Design review of the part built by this model. Coordinates are the model's own, in mm. Coordinates: 2 decimals unless noted, no trailing zeros. Loops run counter-clockwise (first coordinate to the right, second up) from the corner with the lowest first, then second, coordinate; pieces in that order, holes last. Notation, with made-up numbers: M 12,89 L 21,89 A19 cw 21,112 Z; hole C 37.5,-6.75 d8. An arc over 180 degrees is marked long. Write item = value, one per line. Start each with the question number.
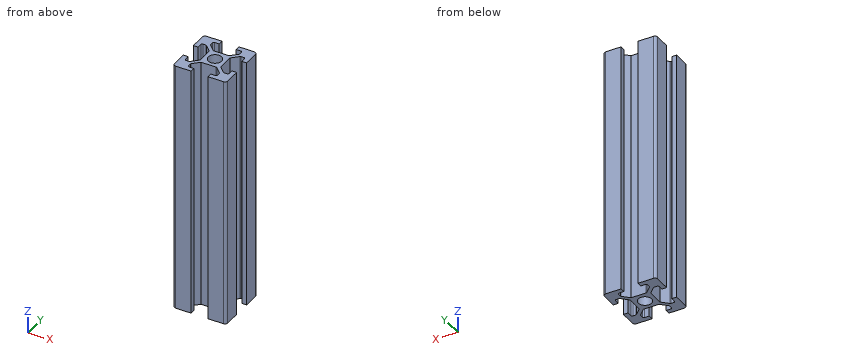
```python
from build123d import *

# Parameters (mm, degrees)
SKETCH1_R           = 2.5
BOSS_EXTRUDE1_DEPTH = 95
FILLET1_R           = 1
FILLET2_R           = 0.5
FILLET3_R           = 0.5
FILLET4_R           = 0.5
FILLET5_R           = 0.5


with BuildPart() as part:
    # Sketch1 → Boss-Extrude1 (new body)
    with BuildSketch(Plane.XY):
        Polygon((13.2, 0), (13.2, 1.8), (15.45, 1.8), (15.45, 3.6), (12.95, 6.1), (7.05, 6.1), (4.55, 3.6), (4.55, 1.8), (6.8, 1.8), (6.8, 0), (0, 0), (0, 6.8), (1.8, 6.8), (1.8, 4.55), (3.6, 4.55), (6.1, 7.05), (6.1, 12.95), (3.6, 15.45), (1.8, 15.45), (1.8, 13.2), (0, 13.2), (0, 20), (6.8, 20), (6.8, 18.2), (4.55, 18.2), (4.55, 16.4), (7.05, 13.9), (12.95, 13.9), (15.45, 16.4), (15.45, 18.2), (13.2, 18.2), (13.2, 20), (20, 20), (20, 13.2), (18.2, 13.2), (18.2, 15.45), (16.4, 15.45), (13.9, 12.95), (13.9, 7.05), (16.4, 4.55), (18.2, 4.55), (18.2, 6.8), (20, 6.8), (20, 0), align=None)
        with Locations((10, 10)):
            Circle(SKETCH1_R, mode=Mode.SUBTRACT)
    extrude(amount=BOSS_EXTRUDE1_DEPTH)

    # Fillet1
    fillet1_edges = [part.edges().sort_by_distance(p)[0] for p in [
        (0, 0, 47.5),
        (0, 20, 47.5),
        (20, 20, 47.5),
        (20, 0, 47.5),
    ]]
    fillet(fillet1_edges, radius=FILLET1_R)

    # Fillet2
    fillet2_edges = [part.edges().sort_by_distance(p)[0] for p in [
        (4.55, 18.2, 47.5),
        (4.55, 16.4, 47.5),
        (7.05, 13.9, 47.5),
        (12.95, 13.9, 47.5),
        (15.45, 16.4, 47.5),
        (15.45, 18.2, 47.5),
    ]]
    fillet(fillet2_edges, radius=FILLET2_R)

    # Fillet3
    fillet3_edges = [part.edges().sort_by_distance(p)[0] for p in [
        (18.2, 15.45, 47.5),
        (16.4, 15.45, 47.5),
        (13.9, 12.95, 47.5),
        (13.9, 7.05, 47.5),
        (16.4, 4.55, 47.5),
        (18.2, 4.55, 47.5),
    ]]
    fillet(fillet3_edges, radius=FILLET3_R)

    # Fillet4
    fillet4_edges = [part.edges().sort_by_distance(p)[0] for p in [
        (1.8, 4.55, 47.5),
        (3.6, 4.55, 47.5),
        (6.1, 7.05, 47.5),
        (6.1, 12.95, 47.5),
        (3.6, 15.45, 47.5),
        (1.8, 15.45, 47.5),
    ]]
    fillet(fillet4_edges, radius=FILLET4_R)

    # Fillet5
    fillet5_edges = [part.edges().sort_by_distance(p)[0] for p in [
        (15.45, 1.8, 47.5),
        (15.45, 3.6, 47.5),
        (12.95, 6.1, 47.5),
        (7.05, 6.1, 47.5),
        (4.55, 3.6, 47.5),
        (4.55, 1.8, 47.5),
    ]]
    fillet(fillet5_edges, radius=FILLET5_R)


solid = part.part
```
(1) To check wall thickness, follow L1, parallel to X at y = 17.5, z = 51; L2, parallel to Y at x = 10, z = 24; L3, parallel to Y at x = 1, z = 35.5. State the ranges of each line that lie inside material, in increasing order.
(2) Insertion check: pin 1 (2 mm diameter, centred on x = 16.5, y = 10.5, fed in from +Z); pin 2 (0.5 mm diameter, centred on y = 19.5, z = 40, fed in from -X). Each pin has a flat end and moves straight along its axis. Give the tip position at first contact, or say it passes through.
(3) Take a section at B-B (x = 8.5). State the section outline as (y, z) points.
(4) Take a section at A-A (y = 10). State the section outline as (x, z) points.
Results list:
q1.L1 = 0 to 4.55, 15.45 to 20
q1.L2 = 6.1 to 7.5, 12.5 to 13.9
q1.L3 = 0 to 6.8, 13.2 to 20
q2.pin_1 = through
q2.pin_2 = 0.03
q3.outline = M 6.1,0 L 8,0 L 8,95 L 6.1,95 Z; M 12,0 L 13.9,0 L 13.9,95 L 12,95 Z
q4.outline = M 6.1,0 L 7.5,0 L 7.5,95 L 6.1,95 Z; M 12.5,0 L 13.9,0 L 13.9,95 L 12.5,95 Z
